from build123d import *

# Parameters (mm, degrees)
CROQUIS1_W              = 60
CROQUIS1_H              = 60
SALIENTE_EXTRUIR1_DEPTH = 20
SALIENTE_EXTRUIR2_DEPTH = 20
CROQUIS3_W              = 20
CROQUIS3_H              = 20
SALIENTE_EXTRUIR3_DEPTH = 20


with BuildPart() as part:
    # Croquis1 → Saliente-Extruir1 (new body)
    with BuildSketch(Plane(origin=(0, 0, 0), x_dir=(1, 0, 0), z_dir=(0, 1, 0))):
        Rectangle(CROQUIS1_W, CROQUIS1_H)
    extrude(amount=SALIENTE_EXTRUIR1_DEPTH)

    # Croquis2 → Saliente-Extruir2 (add)
    with BuildSketch(Plane(origin=(0, 20, 0), x_dir=(1, 0, 0), z_dir=(0, 1, 0))):
        Polygon((-30, -30), (-10, -30), (-10, 10), (10, 10), (10, 30), (-30, 30), align=None)
    extrude(amount=SALIENTE_EXTRUIR2_DEPTH)

    # Croquis3 → Saliente-Extruir3 (add)
    with BuildSketch(Plane(origin=(0, 40, 0), x_dir=(1, 0, 0), z_dir=(0, 1, 0))):
        with Locations((-20, -20)):
            Rectangle(CROQUIS3_W, CROQUIS3_H)
    extrude(amount=SALIENTE_EXTRUIR3_DEPTH)


solid = part.part
Read the model definition and answer for the solid it produces. Units are mm, in the model's axes. A direction names the side the tool comes from. Round coordinates to 2 decimals unless told otherwise and drop trailing zeros. Order: outer loops, then holes, each group sorted by start corner. A loop starts at its lowest first (then second) coordinate and runs counter-clockwise, first axis right, second up. Notation, with made-up numbers: (22, 64) - (28, 64) arc R11 cw to (28, 74) - close; hole circle Ø7 at (-39.75, -39.75). An arc over 180 degrees is marked (long way). Use one line per item in the form item = value. Start each with the question number.
(1) The part is cut by section C-C (y = 54.5). Give the vertices of the cut face in (x, z), then the cut area to 3 significant figures.
(2) The part is cut by section A-A (y = 27.5). Give the vertices of the cut face in (x, z), then the cut area to 3 significant figures.
(3) The part is cut by section B-B (x = 7.5). Give the vertices of the cut face in (y, z).
(4) For faces 1 (the face through (0, 30, -10)), 2 (the face through (-6, 20, -30)), 3 (the face through (10, 30, -20)), 4 (the face through (-20, 50, 10)), determine the directions among +Z, -Z, +X, -X, +Y, -Y from which every point of the face is accessible in a straight line to the end or side of a thin tool.
(5) Flat-ended cylindrical pins translate along their axes: pin 1 Ø16 at (x, y) = (-22.5, 48.5) entering from -Z; pin 2 Ø16 at (x, y) = (2, 32.5) entering from +Z; pin 3 Ø10 at (x, z) = (-1, 0) entering from +Y. Find the tip coordinate at first contact, or state that the pin passes through.
(6) Find the intervals of material crossed by line 1 along Y through (x, z) = (-2, -6); line 2 along X through (y, z) = (28, -9); line 3 along Z through (x, y) = (-16.5, 45), in increasing order. Write a range as from..to.
Checked values:
q1.outline = (-30, 10) - (-10, 10) - (-10, 30) - (-30, 30) - close
q1.area = 400 mm^2
q2.outline = (-30, -30) - (10, -30) - (10, -10) - (-10, -10) - (-10, 30) - (-30, 30) - close
q2.area = 1,600 mm^2
q3.outline = (0, -30) - (40, -30) - (40, -10) - (20, -10) - (20, 30) - (0, 30) - close
q4.face_1 = +Z, +X, +Y
q4.face_2 = -Z, +X, -X, +Y, -Y
q4.face_3 = +Z, -Z, +X, +Y
q4.face_4 = -Z, +X, -X, +Y
q5.pin_1 = 10
q5.pin_2 = -10
q5.pin_3 = 20
q6.line_1 = 0..20
q6.line_2 = -30..-10
q6.line_3 = 10..30
